Here's how the part is built. I have some questions about the finished solid (model axes, mm). Coordinates: 2 decimals unless noted, no trailing zeros. Loops run counter-clockwise (first coordinate to the right, second up) from the corner with the lowest first, then second, coordinate; pieces in that order, holes last. Notation, with made-up numbers: (-7.5, 10.5) - (20.5, 10.5) arc R15 ccw to (20.5, 38.5) - close; hole circle Ø11 at (75.5, -39). An arc over 180 degrees is marked (long way). Use a Markdown table: item, result.
```python
from build123d import *

# Parameters (mm, degrees)
SKETCH1_RX          = 380
SKETCH1_RY          = 290
BOSS_EXTRUDE1_DEPTH = 10
BOSS_EXTRUDE2_DEPTH = 10
CUT_EXTRUDE1_DEPTH  = 10
SKETCH8_W           = 355.795250099
SKETCH8_H           = 262.515596516
CUT_EXTRUDE2_DEPTH  = 102.013832803


with BuildPart() as part:
    # Sketch1 → Boss-Extrude1 (new body)
    with BuildSketch(Plane(origin=(0, 0, 0), x_dir=(1, 0, 0), z_dir=(0, 1, 0))):
        with Locations(Location((0, 0), (0, 0, 90))):
            Ellipse(SKETCH1_RX, SKETCH1_RY)
    extrude(amount=BOSS_EXTRUDE1_DEPTH)

    # Sketch2 → Boss-Extrude2 (add)
    with BuildSketch(Plane(origin=(0, 10, 0), x_dir=(1, 0, 0), z_dir=(0, 1, 0))):
        Polygon((287.228032818, 98.993347022), (277.229646496, 95.262936552), (290, 0), (296.597160239, 102.488980208), align=None)
        Polygon((-296.597160239, 102.488980208), (-290, 0), (-277.229646496, 95.262936552), (-287.228032818, 98.993347022), align=None)
        Polygon((244.797124663, 227.718261487), (188.989530622, 288.225103524), (257.336277473, 164.50388217), (262.120047497, 166.288712763), (271.489174918, 169.784345949), (266.534927877, 209.025181731), align=None)
        Polygon((-266.534927877, 209.025181731), (-271.489174918, 169.784345949), (-262.120047497, 166.288712763), (-257.336277473, 164.50388217), (-188.989530622, 288.225103524), (-244.797124663, 227.718261487), align=None)
    extrude(amount=-BOSS_EXTRUDE2_DEPTH)

    # Sketch4 → Cut-Extrude1 (cut)
    with BuildSketch(Plane(origin=(256.485650454, 95.695117721, -95.695117721), x_dir=(-0.309165432, -0.11535001, -0.943986817), z_dir=(0.884433277, 0.329983165, -0.329983165))):
        Polygon((4.647435865, -100.404384349), (0.972491464, -70.555212825), (72.260950701, -61.778382153), (74.730936612, -81.840463395), (75.935895102, -91.627553677), align=None)
    cut_extrude1 = extrude(amount=-CUT_EXTRUDE1_DEPTH, mode=Mode.SUBTRACT)

    # Mirror1: Cut-Extrude1 across plane
    add(cut_extrude1.mirror(Plane(origin=(0, 0, 0), x_dir=(0, 0, 1), z_dir=(1, 0, 0))), mode=Mode.SUBTRACT)

    # Sketch8 → Cut-Extrude2 (cut, through all)
    with BuildSketch(Plane(origin=(256.485650454, 95.695117721, -95.695117721), x_dir=(-0.309165432, -0.11535001, -0.943986817), z_dir=(0.884433277, 0.329983165, -0.329983165))):
        with Locations((60.595009972, -108.189381189)):
            Rectangle(SKETCH8_W, SKETCH8_H)
    cut_extrude2 = extrude(amount=CUT_EXTRUDE2_DEPTH, mode=Mode.SUBTRACT)

    # Mirror2: Cut-Extrude2 across plane
    add(cut_extrude2.mirror(Plane(origin=(0, 0, 0), x_dir=(0, 0, 1), z_dir=(1, 0, 0))), mode=Mode.SUBTRACT)


solid = part.part
```
Q1. I want a section at A-A, the plane z = -267. Write out the boundary of the cut face in (x, y).
Check values:
| item | result |
|---|---|
| outline | (-208.57, 0) - (208.57, 0) - (208.57, 10) - (-208.57, 10) - close |
Q2. Will these pins go through, and if not, where does the flat tip stop? P1, Ø6, axis at x = -102.5, y = 4, coming from the -Z side; P2, Ø5, axis at x = -129.5, y = 4.5, coming from the -Z side; P3, Ø1.5, axis at x = -193.5, y = 7, coming from the +Z side.
Check values:
| item | result |
|---|---|
| P1 | z = -356.93 |
| P2 | z = -341.62 |
| P3 | z = 283.92 |
Q3. If we mould it in two halves opening along Z, with no side actions, what happens to faces 1 (the face through (-266.17, 5.1, -130.03)), 2 (the face through (-4, 0, -5)), 3 (the face through (215.696, 5.07, -259.27)), 4 (the face through (266.17, 5.1, -130.03))? For each: pulls with the +Z half, pulls with the -Z half, needs draft (parallel to the pull), parting line crosses it, or undercut.
Check values:
| item | result |
|---|---|
| face 1 | undercut |
| face 2 | needs draft |
| face 3 | pulls with the -Z half |
| face 4 | undercut |
Q4. I want a section at B-B, the plane z = -182. Write out the boundary of the cut face in (x, y), then the cut area to 3 significant figures.
Check values:
| item | result |
|---|---|
| outline | (-259.99, 0) - (259.99, 0) - (256.26, 10) - (-256.26, 10) - close |
| area | 5,160 mm^2 |
Q5. Please list where these lines run through material, in increasing order: L1, parallel to X at y = 1.5, z = 12; L2, parallel to X at y = 2.5, z = -224.5; L3, parallel to Z at x = 112, y = 8.25. Write a range as from..to.
Check values:
| item | result |
|---|---|
| L1 | -289.86..289.86 |
| L2 | -243.2..243.2 |
| L3 | -350.52..350.52 |
